The model under review builds one solid part; all positions refer to its coordinate system, in mm. A direction names the side the tool comes from. Coordinates: 2 decimals unless noted, no trailing zeros. Order: outer loops, then holes, each group sorted by start corner. A loop starts at its lowest first (then second) coordinate and runs counter-clockwise, first axis right, second up.
```python
from build123d import *

# Parameters (mm, degrees)
SKETCH_1_W                   = 21
SKETCH_1_H                   = 3
EXTRUDE_1_DEPTH              = 1
SKETCH_3_W                   = 3
SKETCH_3_H                   = 21
EXTRUDE_3_DEPTH              = 1
SKETCH_2_R                   = 2.25
EXTRUDE_4_DEPTH              = 2
HOLE_WIZARD_M2_2_D           = 2.2
HOLE_WIZARD_M2_2_CBORE_D     = 4
HOLE_WIZARD_M2_2_CBORE_DEPTH = 0.5


with BuildPart() as part:
    # ｽｹｯﾁ1 → ﾎﾞｽ - 押し出し1 (new body)
    with BuildSketch(Plane(origin=(0, 0, 0), x_dir=(1, 0, 0), z_dir=(0, 1, 0))):
        Rectangle(SKETCH_1_W, SKETCH_1_H)
    extrude(amount=EXTRUDE_1_DEPTH)

    # ｽｹｯﾁ3 → ﾎﾞｽ - 押し出し3 (add)
    with BuildSketch(Plane.XZ):
        with Locations((-10.5, 10.5)):
            Rectangle(SKETCH_3_W, SKETCH_3_H)
    extrude_3 = extrude(amount=-EXTRUDE_3_DEPTH)

    # ｽｹｯﾁ2 → ﾎﾞｽ - 押し出し4 (add)
    with BuildSketch(Plane.XZ):
        with Locations(Location((-10.5, 0, 0), (0, 0, 270))):
            Circle(SKETCH_2_R)
        with Locations(Location((-10.5, 21, 0), (0, 0, 270))):
            Circle(SKETCH_2_R)
    extrude_4 = extrude(amount=-EXTRUDE_4_DEPTH)

    # M2 なべ頭ねじ用座ぐり穴2 (through all)
    with Locations(Plane(origin=(0, 2, 0), x_dir=(1, 0, 0), z_dir=(0, 1, 0))):
        with Locations((-10.5, 0), (-10.5, -21)):
            hole_wizard_m2_2 = CounterBoreHole(HOLE_WIZARD_M2_2_D / 2, HOLE_WIZARD_M2_2_CBORE_D / 2, HOLE_WIZARD_M2_2_CBORE_DEPTH)

    # ﾐﾗｰ2: ﾎﾞｽ - 押し出し3, ﾎﾞｽ - 押し出し4, M2 なべ頭ねじ用座ぐり穴2 across plane
    add(extrude_3.mirror(Plane(origin=(0, 0, 0), x_dir=(0, 0, 1), z_dir=(1, 0, 0))))
    add(extrude_4.mirror(Plane(origin=(0, 0, 0), x_dir=(0, 0, 1), z_dir=(1, 0, 0))))
    add(hole_wizard_m2_2.mirror(Plane(origin=(0, 0, 0), x_dir=(0, 0, 1), z_dir=(1, 0, 0))), mode=Mode.SUBTRACT)


solid = part.part
```
(1) Draft analysis for pull direction X (two halves, no side actions). For faces 1 (the face through (-12, 0.5, 10.4)), 2 (the face through (-1, 0, 1)), 3 (the face through (10.262, 0.74, 22.074)), state which applies: released by +X, released by -X, zero draft, split by the parting line, or undercut.
A:
face 1: released by -X
face 2: zero draft
face 3: undercut
(2) We need section C-C, the plane x = -10.5. Write out the cut boundary in (y, z), and give its area (3 significant figures).
A:
outline: (0, -2.25) - (2, -2.25) - (2, -2) - (1.5, -2) - (1.5, -1.1) - (0, -1.1) - close; (0, 1.1) - (1.5, 1.1) - (1.5, 2) - (2, 2) - (2, 2.25) - (1, 2.25) - (1, 18.75) - (2, 18.75) - (2, 19) - (1.5, 19) - (1.5, 19.9) - (0, 19.9) - close; (0, 22.1) - (1.5, 22.1) - (1.5, 23) - (2, 23) - (2, 23.25) - (0, 23.25) - close
area: 23.9 mm2
(3) Machinability: for faces 4 (the face through (-0.1, 0.5, -1.5)), 5 (the face through (12.1, 1.8, 1.2)), 6 (the face through (9, 0.5, 10.4)), which of the approach directions +Z, -Z, +X, -X, +Y, -Y give a long, thin tool a straight path to every point of the face, cutting with its end or side? Answer none if there is none.
A:
face 4: -Z, +Y, -Y
face 5: +Y
face 6: +Y, -Y
(4) Wall thickness on probe 1 along X at (y, z) = (1.75, 21); probe 2 along Z at (x, y) = (-10.5, 1.8); probe 3 along Z at (x, y) = (10.5, 0.6): over which ranges is each line inside the solid? List them lowest first.
A:
probe 1: x = -12.75 to -12.5, -8.5 to -8.25, 8.25 to 8.5, 12.5 to 12.75
probe 2: z = -2.25 to -2, 2 to 2.25, 18.75 to 19, 23 to 23.25
probe 3: z = -2.25 to -1.1, 1.1 to 19.9, 22.1 to 23.25
(5) We need section B-B, the plane y = 0.45. Write out the cut boundary in (x, z), and give its area (3 significant figures).
A:
outline: (-12, 1.68) arc R2.25 ccw (long way) to (-8.82, -1.5) - (8.82, -1.5) arc R2.25 ccw (long way) to (12, 1.68) - (12, 19.32) arc R2.25 ccw (long way) to (9, 19.32) - (9, 1.68) arc R2.25 ccw to (8.82, 1.5) - (-8.82, 1.5) arc R2.25 ccw to (-9, 1.68) - (-9, 19.32) arc R2.25 ccw (long way) to (-12, 19.32) - close; hole circle Ø2.2 at (-10.5, 0); hole circle Ø2.2 at (-10.5, 21); hole circle Ø2.2 at (10.5, 0); hole circle Ø2.2 at (10.5, 21)
area: 200 mm2
(6) We need section A-A, the plane z = 21. Write out the cut boundary in (x, y), and give its area (3 significant figures).
A:
outline: (-12.75, 0) - (-11.6, 0) - (-11.6, 1.5) - (-12.5, 1.5) - (-12.5, 2) - (-12.75, 2) - close; (-9.4, 0) - (-8.25, 0) - (-8.25, 2) - (-8.5, 2) - (-8.5, 1.5) - (-9.4, 1.5) - close; (8.25, 0) - (9.4, 0) - (9.4, 1.5) - (8.5, 1.5) - (8.5, 2) - (8.25, 2) - close; (11.6, 0) - (12.75, 0) - (12.75, 2) - (12.5, 2) - (12.5, 1.5) - (11.6, 1.5) - close
area: 7.40 mm2
(7) We need section D-D, the plane z = 11.75. Write out the cut boundary in (x, y), and give its area (3 significant figures).
A:
outline: (-12, 0) - (-9, 0) - (-9, 1) - (-12, 1) - close; (9, 0) - (12, 0) - (12, 1) - (9, 1) - close
area: 6.00 mm2
(8) For pin 1 Ø0.9 at (x, z) = (10, 13.5) entering from +Y; pin 2 Ø3.5 at (x, z) = (10.5, 0) entering from +Y; pin 3 Ø0.5 at (x, y) = (-4, 0.5) entering from -Z, all flat-tipped, find the tip position at first contact; note any pin that passes through.
A:
pin 1: stops at y = 1
pin 2: stops at y = 1.5
pin 3: stops at z = -1.5
